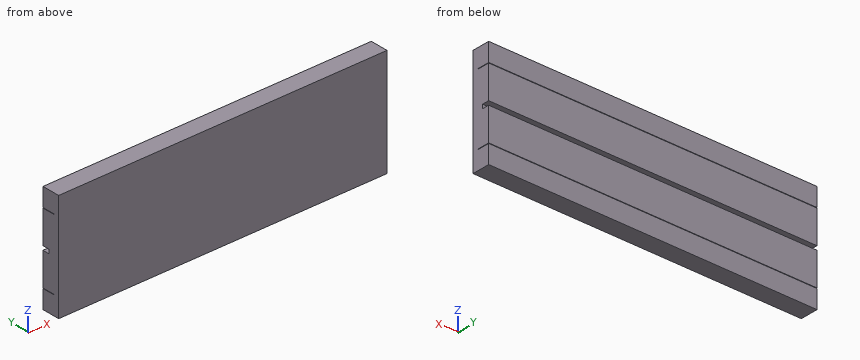
Autodesk Inventor part; units mm, degrees
ref_plane "YZ Plane" through (0, 0, 0) normal (1, 0, 0) x (0, 1, 0)
ref_plane "XZ Plane" through (0, 0, 0) normal (0, 1, 0) x (-1, 0, 0)
ref_plane "XY Plane" through (0, 0, 0) normal (0, 0, 1) x (1, 0, 0)
sketch "Sketch1" plane through (0, 0, 0) normal (0, 1, 0) x (-1, 0, 0)
  line L0 (82.5, -27) -> (-82.5, -27)
  line L1 (-82.5, -27) -> (-82.5, 27)
  line L2 (-82.5, 27) -> (82.5, 27)
  line L3 (82.5, 27) -> (82.5, -27)
  line L4 (82.5, -27) -> (-82.5, 27) construction
  line L5 (-82.5, -27) -> (82.5, 27) construction
  point P0 (0, 0)
  dimension "d0" = 165
  dimension "d1" = 54
extrude "Extrusion1" add sketch "Sketch1" along normal blind 9
sketch "Sketch2" plane through (82.5, 0, 27) normal (1, 0, 0) x (0, 0, -1)
  line L0 (0, 9) -> (54, 9)
  line L1 (27, 0) -> (27, 9) construction
  line L2 (26, 12.517) -> (28, 12.517)
  line L3 (28, 12.517) -> (28, 5.483)
  line L4 (28, 5.483) -> (26, 5.483)
  line L5 (26, 5.483) -> (26, 12.517)
  line L6 (26, 12.517) -> (28, 5.483) construction
  line L7 (28, 12.517) -> (26, 5.483) construction
  dimension "d4" = 2
extrude "Extrusion2" cut sketch "Sketch2" against normal blind 203.725
sketch "Sketch3" plane through (82.5, 0, 27) normal (1, 0, 0) x (0, 0, -1)
  line L0 (27, 0) -> (27, 5.483) construction
  line L1 (28, 5.483) -> (26, 5.483) construction
  line L2 (27, 2.7415) -> (44.5, 2.7415) construction
  line L3 (44.5, 2.7415) -> (44.75, 2.7415)
  line L4 (44.75, 2.7415) -> (44.75, 10.8697)
  line L5 (44.75, 10.8697) -> (44.5, 10.8697)
  line L6 (44.5, 10.8697) -> (44.5, 2.7415)
  line L7 (9.5, 2.7415) -> (9.25, 2.7415)
  line L8 (9.25, 2.7415) -> (9.25, 10.8697)
  line L9 (9.25, 10.8697) -> (9.5, 10.8697)
  line L10 (9.5, 10.8697) -> (9.5, 2.7415)
  dimension "d7" = 17.5
  dimension "d8" = 0.25
extrude "Extrusion3" cut sketch "Sketch3" against normal blind 203.725
properties part number "Large Bread Board" material "PC/ABS Plastic"
Geometry: final body of the model. Coordinates: model frame, mm. Coordinates: 2 decimals unless noted, no trailing zeros. Order: outer loops, then holes, each group sorted by start corner. A loop starts at its lowest first (then second) coordinate and runs counter-clockwise, first axis right, second up. Notation, with made-up numbers: (44.5, -17) -> (93.5, -17) arc R32 cw to (93.5, 17) -> close; hole circle Ø9 at (46.5, -27). An arc over 180 degrees is marked (long way). Use CSV: the item, a comma, the result in double quotes.
1) Section B-B on x = 68. Output: boundary loops of the cut face in (y, z).
Findings:
outline,"(0, -27) -> (9, -27) -> (9, -17.75) -> (2.74, -17.75) -> (2.74, -17.5) -> (9, -17.5) -> (9, -1) -> (5.48, -1) -> (5.48, 1) -> (9, 1) -> (9, 17.5) -> (2.74, 17.5) -> (2.74, 17.75) -> (9, 17.75) -> (9, 27) -> (0, 27) -> close"
2) Line query: line 1 (Z direction, x = 67.5, y = 5.75); line 2 (Z direction, x = -67.5, y = 5.25); line 3 (Y direction, x = -59, z = 0). Output: solid intervals per line, ascending.
Findings:
line 1,"z = -27 to -17.75, -17.5 to -1, 1 to 17.5, 17.75 to 27"
line 2,"z = -27 to -17.75, -17.5 to 17.5, 17.75 to 27"
line 3,"y = 0 to 5.48"
3) Section A-A on y = 7.25. Output: boundary loops of the cut face in (x, z), then the cut area to 3 significant figures.
Findings:
outline,"(-82.5, -27) -> (82.5, -27) -> (82.5, -17.75) -> (-82.5, -17.75) -> close; (-82.5, -17.5) -> (82.5, -17.5) -> (82.5, -1) -> (-82.5, -1) -> close; (-82.5, 1) -> (82.5, 1) -> (82.5, 17.5) -> (-82.5, 17.5) -> close; (-82.5, 17.75) -> (82.5, 17.75) -> (82.5, 27) -> (-82.5, 27) -> close"
area,"8,500 mm^2"
